from build123d import *

# Parameters (mm, degrees)
F0_W      = 52.3
F0_H      = 52.3
F1_DEPTH  = 5
F3_DEPTH  = 5
F4_W      = 52.3
F4_H      = 55
F5_DEPTH  = 20
F7_DEPTH  = 52.3
F8_R      = 5
F8_R_2    = 4.357139
F9_DEPTH  = 50
F10_R     = 2.5
F11_DEPTH = 55.001
F13_DEPTH = 52.3
F14_W     = 52.3
F14_H     = 5
F15_DEPTH = 70
F17_DEPTH = 89.648963
F18_R     = 10
F19_R     = 12.5
F19_R_2   = 1.5
F20_DEPTH = 5.001
F21_R     = 2.5
F22_DEPTH = 25.001


with BuildPart() as f1:
    # F0 (on Top) → F1 (new body)
    with BuildSketch(Plane.XY):
        with Locations((26.15, 26.15)):
            Rectangle(F0_W, F0_H)
    extrude(amount=F1_DEPTH)

    # F2 (on Right) → F3 (join)
    with BuildSketch(Plane.YZ):
        Polygon((0, 0), (52.3, 0), (87.273074, 75), (26.15, 75), (-34.973074, 75), align=None)
    extrude(amount=-F3_DEPTH)

    # F4 (on face) → F5 (join)
    with BuildSketch(Plane(origin=(-5, 0, 0), x_dir=(0, -1, 0), z_dir=(-1, 0, 0))):
        with Locations((-26.15, 27.5)):
            Rectangle(F4_W, F4_H)
    extrude(amount=F5_DEPTH)

    # F6 (on face) → F7 (cut, through all)
    with BuildSketch(Plane(origin=(0, 52.3, 0), x_dir=(-1, 0, 0), z_dir=(0, 1, 0))):
        Polygon((25, 55), (5, 0), (25, 0), align=None)
    extrude(amount=-F7_DEPTH, mode=Mode.SUBTRACT)

    # F8 (on Top) → F9 (cut)
    with BuildSketch(Plane.XY):
        with Locations((-15, 10)):
            Circle(F8_R)
        with Locations((-15, 42.3)):
            Circle(F8_R_2)
    extrude(amount=F9_DEPTH, mode=Mode.SUBTRACT)

    # F10 (on face) → F11 (cut, through all)
    with BuildSketch(Plane.XY.offset(55)):
        with Locations((-15, 42.3)):
            Circle(F10_R)
        with Locations((-15, 10)):
            Circle(F10_R)
    extrude(amount=-F11_DEPTH, mode=Mode.SUBTRACT)

    # F12 (on face) → F13 (join, through all)
    with BuildSketch(Plane.YZ.offset(52.3)):
        Polygon((0, 0), (0, 5), (-2.374889, 5), align=None)
        Polygon((54.674889, 5), (52.3, 5), (52.3, 0), align=None)
    extrude(amount=-F13_DEPTH)

    # F14 (on face) → F15 (join, through all)
    with BuildSketch(Plane.XY.offset(5)):
        with Locations((26.15, 52.174889)):
            Rectangle(F14_W, F14_H)
        with Locations((26.15, 0.125111)):
            Rectangle(F14_W, F14_H)
    extrude(amount=F15_DEPTH)

    # F16 (on face) → F17 (cut, through all)
    with BuildSketch(Plane.XZ.offset(2.374889)):
        Polygon((52.3, 75), (0, 75), (52.3, 5), align=None)
    extrude(amount=-F17_DEPTH, mode=Mode.SUBTRACT)

    # F18
    f18_edges = [f1.edges().sort_by_distance(p)[0] for p in [
        (-2.5, -34.973074, 75),
        (-2.5, 87.273074, 75),
    ]]
    fillet(f18_edges, radius=F18_R)

    # F19 (on face) → F20 (cut, through all)
    with BuildSketch(Plane.XY.offset(5)):
        with Locations((26.15, 26.15)):
            Circle(F19_R)
        with Locations((4.72885, 6.879248)):
            Circle(F19_R_2)
        with Locations((4.72885, 45.420752)):
            Circle(F19_R_2)
        with Locations((47.57115, 45.420752)):
            Circle(F19_R_2)
        with Locations((47.57115, 6.879248)):
            Circle(F19_R_2)
    extrude(amount=-F20_DEPTH, mode=Mode.SUBTRACT)

    # F21 (on face) → F22 (cut, through all)
    with BuildSketch(Plane.YZ):
        with Locations((-19.276219, 65)):
            Circle(F21_R)
        with Locations((71.576219, 65)):
            Circle(F21_R)
    extrude(amount=-F22_DEPTH, mode=Mode.SUBTRACT)


solid = f1.part
Can you work these out from the model? Positions are in its coordinate system, mm. A direction names the side the tool comes from. Round coordinates to 2 decimals unless told otherwise and drop trailing zeros. Write each loop counter-clockwise with the first axis right and the second up, starting at its lowest first coordinate (ties: lowest second). Pieces come first, ordered by that corner, then holes. Notation, with made-up numbers: (-3, 38.5) - (38, 38.5) arc R26 cw to (38, 77.5) - close; hole circle Ø7 at (-32, 55.25). An arc over 180 degrees is marked (long way). Write each question's results on one line, items separated by ' | '. Start each with the question number.
1) Suppose I cut it at C-C (x = 26.15). List the corners of the cut face in (y, z) for me, and give its area (3 significant figures).
2) Suppose I cut it at A-A (y = 10). List the corners of the cut face in (x, z) for me, and give its area (4 significant figures).
3) For pin 1 Ø2 at (x, z) = (-7.5, 62) entering from +Y; pin 2 Ø6 at (y, z) = (27, 12) entering from +X; pin 3 Ø10 at (x, y) = (39.5, 10) entering from +Z; pin 4 Ø6 at (x, y) = (-17, 15.5) entering from +Z, each with a flat end and sliding along its axis, tell me the tip position at first contact or that it passes through.
4) Which directions (+Z, -Z, +X, -X, +Y, -Y) give clear straight access to the entire face, cutting with the end or side of a thin tool? Please do faces 4 (the flat face through (-10, 52.3, 39)), 5 (the flat face through (-10, 0, 39)), 6 (the flat face through (20, -2.375, 32)), 7 (the flat face through (38, 32, 5)).
5) Suppose I cut it at D-D (y = 26.15). List the corners of the cut face in (x, z) for me.
6) Please list where these lines run through material, in increasing order: line 1 (Y direction, x = -14.5, z = 46); line 2 (Y direction, x = -15, z = 52.7); line 3 (Y direction, x = 21.5, z = 31.5).
7) Suppose I cut it at B-B (x = -15). List the corners of the cut face in (y, z) for me, and give its area (3 significant figures).
8) We'd pull the mould along X, two halves only. Please class faces 1 (the cylindrical face through (-2.535, 80.085, 70.254)), 2 (the flat face through (-15.14, 26.52, 27.88)), 3 (the cylindrical face through (48.26, 44.09, 2.54)): released by +X, released by -X, zero draft, split by the parting line, or undercut.
Here are the results:
1) outline: (-2.37, 5) - (0, 0) - (13.65, 0) - (13.65, 5) - (2.63, 5) - (2.63, 40) - (-2.37, 40) - close; (38.65, 0) - (52.3, 0) - (54.67, 5) - (54.67, 40) - (49.67, 40) - (49.67, 5) - (38.65, 5) - close | area: 498 mm2
2) outline: (-25, 55) - (-20, 41.25) - (-20, 50) - (-17.5, 50) - (-17.5, 55) - close; (-12.5, 50) - (-10, 50) - (-10, 13.75) - (-5, 0) - (52.3, 0) - (52.3, 5) - (0, 5) - (0, 75) - (-5, 75) - (-5, 55) - (-12.5, 55) - close | area: 936.5 mm2
3) pin 1: passes through | pin 2: stops at x = 0 | pin 3: stops at z = 5 | pin 4: stops at z = 55
4) face 4: +Z, -Z, -X, +Y | face 5: +Z, -Z, -X, -Y | face 6: +Z, -Z, +X, -Y | face 7: +Z, +X
5) outline: (-25, 55) - (-5, 0) - (13.65, 0) - (13.65, 5) - (0, 5) - (0, 75) - (-5, 75) - (-5, 55) - close; (38.65, 0) - (52.3, 0) - (52.3, 5) - (38.65, 5) - close
6) line 1: y = 0 to 5.03, 14.97 to 37.97, 46.63 to 52.3 | line 2: y = 0 to 7.5, 12.5 to 39.8, 44.8 to 52.3 | line 3: y = -2.37 to 2.63, 49.67 to 54.67
7) outline: (0, 27.5) - (5, 27.5) - (5, 50) - (7.5, 50) - (7.5, 55) - (0, 55) - close; (12.5, 50) - (15, 50) - (15, 27.5) - (37.94, 27.5) - (37.94, 50) - (39.8, 50) - (39.8, 55) - (12.5, 55) - close; (44.8, 50) - (46.66, 50) - (46.66, 27.5) - (52.3, 27.5) - (52.3, 55) - (44.8, 55) - close | area: 967 mm2
8) face 1: zero draft | face 2: released by -X | face 3: undercut
